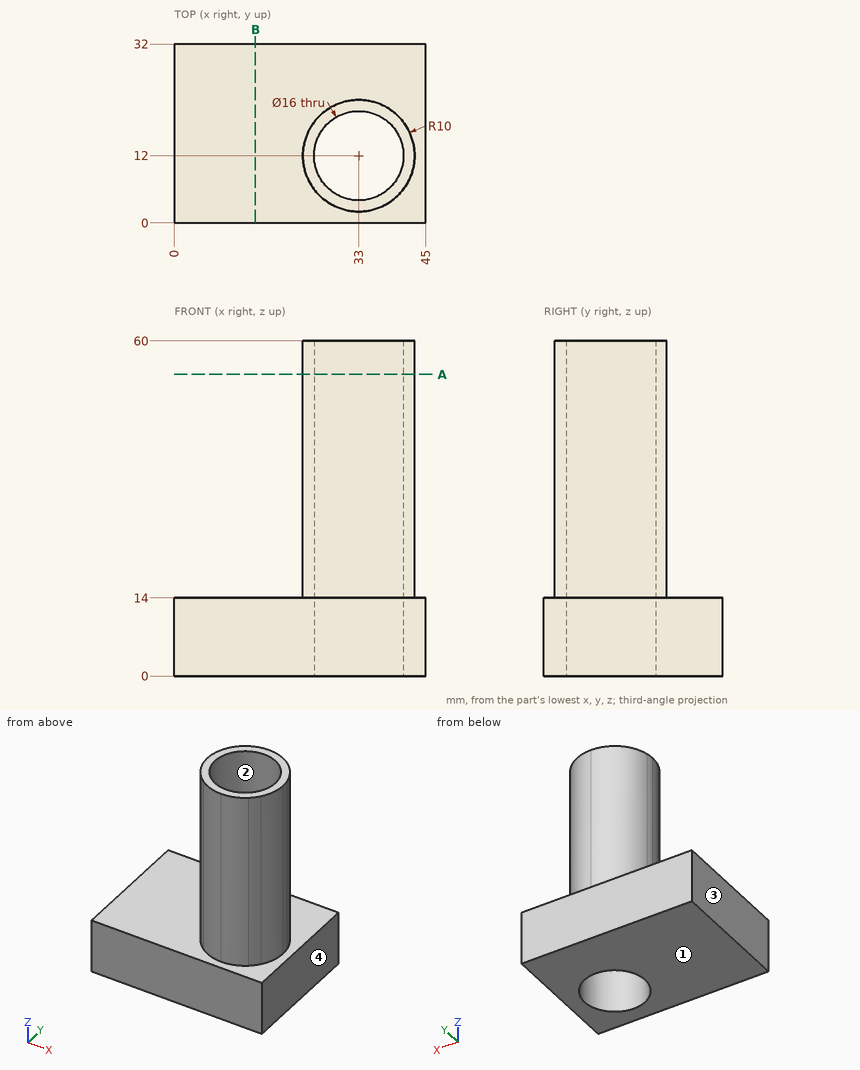
Answer from the drawing. Dimensions are ordinates in mm from the lowest x, y and z of the part. Give positions to 0.01 mm unless a question says otherwise; leave off trailing zeros. Write each loop counter-clockwise with the first axis right and the second up, starting at its lowest first coordinate (ties: lowest second). Pieces come first, ordered by that corner, then holes. Notation, with made-up numbers: (-12, 54) -> (-1, 54) arc R32 cw to (-1, 82) -> close; hole circle Ø4 at (37, 18.25). An arc over 180 degrees is marked (long way). One line per question, with ' | ' between items. Start each with the question number.
1. Given pin 1 Ø3 at (x, y) = (13.5, 27) entering from -Z; pin 2 Ø4 at (x, z) = (32.5, 21) entering from -Y; pin 3 Ø10 at (y, z) = (13, 21.5) entering from -X; pin 4 Ø12 at (y, z) = (17, 35.5) entering from +X, each flat-ended and moving along its own axis, determine where each tip first touches the part or whether it passes through.
2. Section A-A (z = 54) is taken. Determine the outline of the cut face in (x, y).
3. For a pull along X with two mould halves and no side action, classify the marked faces 1, 2, 3 and 4 as pulls with the +X half, pulls with the -X half, needs draft (parallel to the pull), parting line crosses it, or undercut.
4. Find the intervals of material crossed by probe 1 along Y at (x, z) = (33, 41); probe 2 along X at (y, z) = (12, 38.5); probe 3 along X at (y, z) = (12, 12), in increasing order.
5. Section B-B (x = 14.5) is taken. Determine the outline of the cut face in (y, z).
Response values:
1) pin 1: z = 0 | pin 2: y = 2 | pin 3: x = 23 | pin 4: x = 43
2) outline: circle Ø20 at (33, 12); hole circle Ø16 at (33, 12)
3) face 1: needs draft | face 2: undercut | face 3: pulls with the -X half | face 4: pulls with the +X half
4) probe 1: 2 to 4, 20 to 22 | probe 2: 23 to 25, 41 to 43 | probe 3: 0 to 25, 41 to 45
5) outline: (0, 0) -> (32, 0) -> (32, 14) -> (0, 14) -> close
